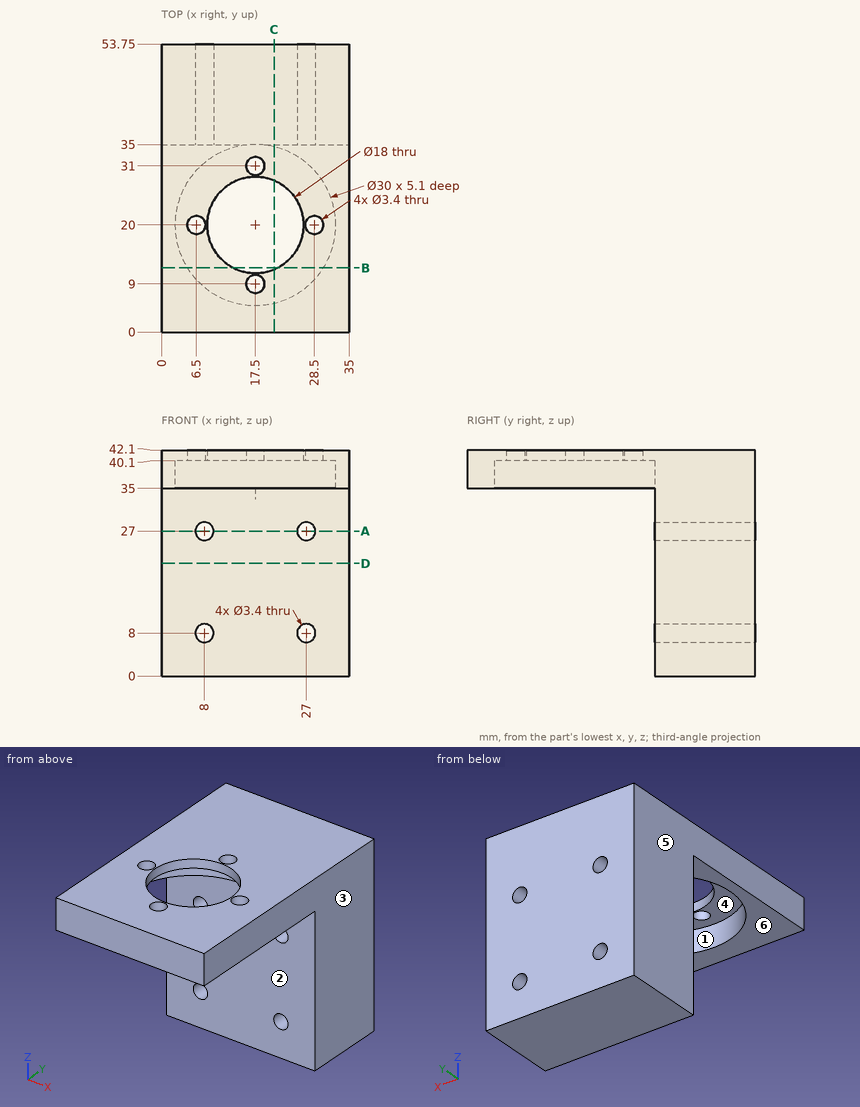
Here's the drawing with two shaded views (mm, measured from the low corner). I have some questions. A direction names the side the tool comes from. Coordinates: 2 decimals unless noted, no trailing zeros. Write each loop counter-clockwise with the first axis right and the second up, starting at its lowest first coordinate (ties: lowest second). Pieces come first, ordered by that corner, then holes. Notation, with made-up numbers: (12.25, 85) -> (32.25, 85) arc R32 ccw to (32.25, 115) -> close; hole circle Ø5 at (39.25, -7.75). An arc over 180 degrees is marked (long way). Answer as CSV lines item,"result".
1) On a 3-axis mill with a long thin cutter (end or side, diameter ignored), from which of +Z, -Z, +X, -X, +Y, -Y can I reach the whole of each face in a straight line? I mean the marked faces 4, 5 and 6. Say none if no direction works.
Check result:
face 4,"-Z"
face 5,"+Z, -Z, -X, +Y, -Y"
face 6,"-Z, +X, -X, -Y"
2) Will these pins go through, and if not, where does the flat tip stop? P1, Ø4.5, axis at x = 28.5, y = 20, coming from the -Z side; P2, Ø17.5, axis at x = 23, z = 26, coming from the -Y side; P3, Ø2, axis at x = 17.5, y = 31, coming from the +Z side.
Check result:
P1,"z = 40.1"
P2,"y = 35"
P3,"through"
3) If we section it at A-A on z = 27: Please give me the cut outline in (x, y).
Check result:
outline,"(0, 35) -> (6.3, 35) -> (6.3, 53.75) -> (0, 53.75) -> close; (9.7, 35) -> (25.3, 35) -> (25.3, 53.75) -> (9.7, 53.75) -> close; (28.7, 35) -> (35, 35) -> (35, 53.75) -> (28.7, 53.75) -> close"
4) If we section it at C-C on x = 21: Please give me the cut outline in (y, z), then the cut area to 3 significant figures.
Check result:
outline,"(0, 35) -> (5.41, 35) -> (5.41, 40.1) -> (11.71, 40.1) -> (11.71, 42.1) -> (0, 42.1) -> close; (28.29, 40.1) -> (34.59, 40.1) -> (34.59, 35) -> (35, 35) -> (35, 0) -> (53.75, 0) -> (53.75, 42.1) -> (28.29, 42.1) -> close"
area,"856 mm²"
5) If we section it at B-B on y = 12: Please give me the cut outline in (x, z), then the cut area to 3 significant figures.
Check result:
outline,"(0, 35) -> (4.81, 35) -> (4.81, 40.1) -> (13.38, 40.1) -> (13.38, 42.1) -> (0, 42.1) -> close; (21.62, 40.1) -> (30.19, 40.1) -> (30.19, 35) -> (35, 35) -> (35, 42.1) -> (21.62, 42.1) -> close"
area,"103 mm²"
6) If I drill on line 1 (X direction, y = 20, z = 41.55); line 2 (Y direction, x = 17.5, z = 41.65); line 3 (Y direction, x = 6.5, z = 40.5), over which ranges is the centre line in solid material (lowest first)? Write a range as from..to.
Check result:
line 1,"0..4.8, 8.2..8.5, 26.5..26.8, 30.2..35"
line 2,"0..7.3, 10.7..11, 29..29.3, 32.7..53.75"
line 3,"0..18.3, 21.7..53.75"
7) If we mould it in two halves opening along X, with no side actions, what happens to the marked faces 1, 2 and 3? For each: +X half, -X half, draft (parallel to the pull), parting line (faces both ways), or undercut.
Check result:
face 1,"undercut"
face 2,"draft"
face 3,"+X half"
8) If we section it at D-D on z = 21: Please give me the cut outline in (x, y).
Check result:
outline,"(0, 35) -> (35, 35) -> (35, 53.75) -> (0, 53.75) -> close"
